Autodesk Inventor part; units mm, degrees
ref_plane "YZ Plane" through (0, 0, 0) normal (1, 0, 0) x (0, 1, 0)
ref_plane "XZ Plane" through (0, 0, 0) normal (0, 1, 0) x (-1, 0, 0)
ref_plane "XY Plane" through (0, 0, 0) normal (0, 0, 1) x (1, 0, 0)
sketch "Sketch1" plane through (0, 0, 0) normal (0, 1, 0) x (-1, 0, 0)
  line L0 (9.5, -44) -> (-9.5, -44)
  line L1 (-9.5, -44) -> (-9.5, 44)
  line L2 (-9.5, 44) -> (9.5, 44)
  line L3 (9.5, 44) -> (9.5, -44)
  line L4 (9.5, -44) -> (-9.5, 44) construction
  line L5 (-9.5, -44) -> (9.5, 44) construction
  point P0 (0, 0)
  dimension "d0" = 19
  dimension "d1" = 88
extrude "Extrusion1" add sketch "Sketch1" along normal blind 10
fillet "Fillet1" radius 4 1 edges at (9.5, 5, 44)
chamfer "Chamfer1" distance 9.5 angle 45 1 edges at (-9.5, 10, 0)
sketch "Sketch2" plane through (9.5, 0, -44) normal (1, 0, 0) x (0, 0, -1)
  line L0 (0, 0) -> (-50, 0)
  line L1 (-50, 0) -> (-50, 5)
  line L2 (-50, 5) -> (0, 5)
  line L3 (0, 5) -> (0, 0)
  line L4 (-6, 5.5) -> (-44, 5.5)
  line L5 (-44, 5.5) -> (-44, 4.5)
  line L6 (-44, 4.5) -> (-6, 4.5)
  line L7 (-6, 4.5) -> (-6, 5.5)
  line L8 (-6, 5.5) -> (-44, 4.5) construction
  line L9 (-44, 5.5) -> (-6, 4.5) construction
  circle A0 centre (-44, 5) radius 0.5
  circle A1 centre (-6, 5) radius 0.5
  point P0 (-44, 0)
  point P1 (-25, 5)
  dimension "d8" = 50
  dimension "d9" = 5
  dimension "d10" = 38
  dimension "d11" = 1
  dimension "d12" = 1
  dimension "d13" = 1
extrude "Extrusion2" cut sketch "Sketch2" against normal blind 2 contours A1 L7 L2 | L2 L7 A1 | A0 L5 L2 | L2 L5 A0 | L7 A1 L2 | L2 A1 L7 | L5 A0 L2 | L2 A0 L5
properties part number "komatex_senzor"
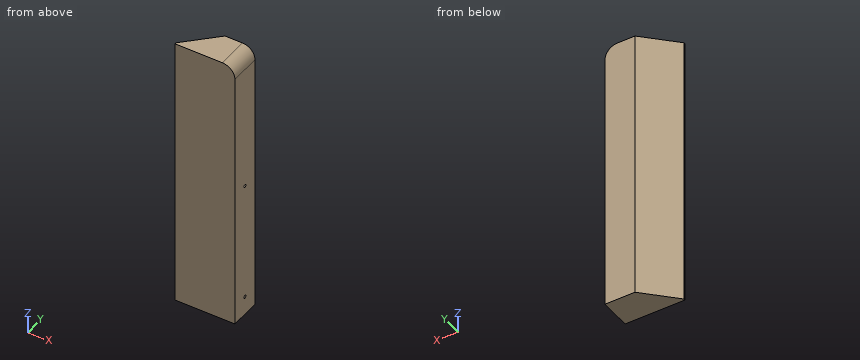
Here's how the part is built. I have some questions about the finished solid (model axes, mm). Round coordinates to 2 decimals unless told otherwise and drop trailing zeros. Write each loop counter-clockwise with the first axis right and the second up, starting at its lowest first coordinate (ties: lowest second). Pieces come first, ordered by that corner, then holes.
1. Will these pins go through, and if not, where does the flat tip stop? pin 1 Ø4 at (x, z) = (-0.5, 18.5) entering from -Y; pin 2 Ø1.5 at (x, z) = (-7, 6.5) entering from +Y; pin 3 Ø0.5 at (y, z) = (5, -38) entering from +X; pin 4 Ø4 at (y, z) = (9, 25) entering from -X.
2. I need wall thicknesses on L1, parallel to Y at x = 9.05, z = -38; L2, parallel to Z at x = 8.6, y = 5; L3, parallel to Z at x = 8.8, y = 5. Which ranges of each line are inside material? Lowest first, please.
3. Suppose I cut it at B-B (z = 9). List the corners of the cut face in (x, y) for me.
4. Suppose I cut it at C-C (x = -3.5). List the corners of the cut face in (y, z) for me.
5. Suppose I cut it at A-A (y = 3.5). List the corners of the cut face in (x, z) for me.
Answer sheet:
1. pin 1: stops at y = 0
1. pin 2: stops at y = 3.75
1. pin 3: stops at x = 7.5
1. pin 4: stops at x = -3
2. L1: y = 0 to 4.5, 5.5 to 10
2. L2: z = -44 to -38.5, -37.5 to -0.5, 0.5 to 42.53
2. L3: z = -44 to -38.5, -37.5 to -0.5, 0.5 to 42.26
3. outline: (-9.5, 0) - (9.5, 0) - (9.5, 10) - (0, 10) - (-9.5, 0.5) - close
4. outline: (0, -44) - (6.5, -44) - (6.5, 44) - (0, 44) - close
5. outline: (-6.5, -44) - (9.5, -44) - (9.5, 40) arc R4 ccw to (5.5, 44) - (-6.5, 44) - close
